```python
from build123d import *

# Parameters (mm, degrees)
F0_R           = 32.5
F0_R_2         = 11.25
F1_DEPTH       = 2
F2_DEPTH       = 2
F3_R           = 32.5
F4_DEPTH       = 2
F6_D           = 3
F6_DEPTH       = 12
F6_CSINK_D     = 6.5
F6_CSINK_ANGLE = 45
F6_TIP         = 0.9012909285


with BuildPart() as f1:
    # F0 (on Top) → F1 (new body)
    with BuildSketch(Plane.XY):
        Circle(F0_R)
        with BuildLine():
            Line((-21.25, 17.4553000547), (-21.25, 21.25))
            Line((-21.25, 21.25), (-17.4553000547, 21.25))
            ThreePointArc((-17.4553000547, 21.25), (0, 27.5), (17.4553000547, 21.25))
            Line((17.4553000547, 21.25), (21.25, 21.25))
            Line((21.25, 21.25), (21.25, 17.4553000547))
            ThreePointArc((21.25, 17.4553000547), (25.8903939715, 9.2702481089), (27.5, 0))
            ThreePointArc((27.5, 0), (25.8903939715, -9.2702481089), (21.25, -17.4553000547))
            Line((21.25, -17.4553000547), (21.25, -21.25))
            Line((21.25, -21.25), (17.4553000547, -21.25))
            ThreePointArc((17.4553000547, -21.25), (0, -27.5), (-17.4553000547, -21.25))
            Line((-17.4553000547, -21.25), (-21.25, -21.25))
            Line((-21.25, -21.25), (-21.25, -17.4553000547))
            ThreePointArc((-21.25, -17.4553000547), (-27.5, 0), (-21.25, 17.4553000547))
        make_face(mode=Mode.SUBTRACT)
        with BuildLine():
            Line((-17.4553000547, 21.25), (-21.25, 21.25))
            Line((-21.25, 21.25), (-21.25, 17.4553000547))
            ThreePointArc((-21.25, 17.4553000547), (-19.4454364826, 19.4454364826), (-17.4553000547, 21.25))
        make_face()
        with BuildLine():
            Line((21.25, 21.25), (17.4553000547, 21.25))
            ThreePointArc((17.4553000547, 21.25), (19.4454364826, 19.4454364826), (21.25, 17.4553000547))
            Line((21.25, 17.4553000547), (21.25, 21.25))
        make_face()
        with BuildLine():
            Line((21.25, -21.25), (21.25, -17.4553000547))
            ThreePointArc((21.25, -17.4553000547), (19.4454364826, -19.4454364826), (17.4553000547, -21.25))
            Line((17.4553000547, -21.25), (21.25, -21.25))
        make_face()
        with BuildLine():
            ThreePointArc((-17.4553000547, -21.25), (-19.4454364826, -19.4454364826), (-21.25, -17.4553000547))
            Line((-21.25, -17.4553000547), (-21.25, -21.25))
            Line((-21.25, -21.25), (-17.4553000547, -21.25))
        make_face()
        with BuildLine():
            Line((17.4553000547, -21.25), (-17.4553000547, -21.25))
            ThreePointArc((-17.4553000547, -21.25), (0, -27.5), (17.4553000547, -21.25))
        make_face()
        with BuildLine():
            ThreePointArc((27.5, 0), (25.8903939715, 9.2702481089), (21.25, 17.4553000547))
            Line((21.25, 17.4553000547), (21.25, -17.4553000547))
            ThreePointArc((21.25, -17.4553000547), (25.8903939715, -9.2702481089), (27.5, 0))
        make_face()
        with BuildLine():
            ThreePointArc((17.4553000547, 21.25), (0, 27.5), (-17.4553000547, 21.25))
            Line((-17.4553000547, 21.25), (17.4553000547, 21.25))
        make_face()
        with BuildLine():
            Line((-21.25, -17.4553000547), (-21.25, 17.4553000547))
            ThreePointArc((-21.25, 17.4553000547), (-27.5, 0), (-21.25, -17.4553000547))
        make_face()
        with BuildLine():
            Line((17.4553000547, 21.25), (-17.4553000547, 21.25))
            ThreePointArc((-17.4553000547, 21.25), (-19.4454364826, 19.4454364826), (-21.25, 17.4553000547))
            Line((-21.25, 17.4553000547), (-21.25, -17.4553000547))
            ThreePointArc((-21.25, -17.4553000547), (-19.4454364826, -19.4454364826), (-17.4553000547, -21.25))
            Line((-17.4553000547, -21.25), (17.4553000547, -21.25))
            ThreePointArc((17.4553000547, -21.25), (19.4454364826, -19.4454364826), (21.25, -17.4553000547))
            Line((21.25, -17.4553000547), (21.25, 17.4553000547))
            ThreePointArc((21.25, 17.4553000547), (19.4454364826, 19.4454364826), (17.4553000547, 21.25))
        make_face()
        Circle(F0_R_2, mode=Mode.SUBTRACT)
    extrude(amount=F1_DEPTH)

    # F0 (on Top) → F2 (join)
    with BuildSketch(Plane.XY):
        Circle(F0_R)
        with BuildLine():
            Line((-21.25, 17.4553000547), (-21.25, 21.25))
            Line((-21.25, 21.25), (-17.4553000547, 21.25))
            ThreePointArc((-17.4553000547, 21.25), (0, 27.5), (17.4553000547, 21.25))
            Line((17.4553000547, 21.25), (21.25, 21.25))
            Line((21.25, 21.25), (21.25, 17.4553000547))
            ThreePointArc((21.25, 17.4553000547), (25.8903939715, 9.2702481089), (27.5, 0))
            ThreePointArc((27.5, 0), (25.8903939715, -9.2702481089), (21.25, -17.4553000547))
            Line((21.25, -17.4553000547), (21.25, -21.25))
            Line((21.25, -21.25), (17.4553000547, -21.25))
            ThreePointArc((17.4553000547, -21.25), (0, -27.5), (-17.4553000547, -21.25))
            Line((-17.4553000547, -21.25), (-21.25, -21.25))
            Line((-21.25, -21.25), (-21.25, -17.4553000547))
            ThreePointArc((-21.25, -17.4553000547), (-27.5, 0), (-21.25, 17.4553000547))
        make_face(mode=Mode.SUBTRACT)
        with BuildLine():
            Line((-21.25, -17.4553000547), (-21.25, 17.4553000547))
            ThreePointArc((-21.25, 17.4553000547), (-27.5, 0), (-21.25, -17.4553000547))
        make_face()
        with BuildLine():
            Line((17.4553000547, -21.25), (-17.4553000547, -21.25))
            ThreePointArc((-17.4553000547, -21.25), (0, -27.5), (17.4553000547, -21.25))
        make_face()
        with BuildLine():
            ThreePointArc((27.5, 0), (25.8903939715, 9.2702481089), (21.25, 17.4553000547))
            Line((21.25, 17.4553000547), (21.25, -17.4553000547))
            ThreePointArc((21.25, -17.4553000547), (25.8903939715, -9.2702481089), (27.5, 0))
        make_face()
        with BuildLine():
            ThreePointArc((17.4553000547, 21.25), (0, 27.5), (-17.4553000547, 21.25))
            Line((-17.4553000547, 21.25), (17.4553000547, 21.25))
        make_face()
        with BuildLine():
            ThreePointArc((-17.4553000547, -21.25), (-19.4454364826, -19.4454364826), (-21.25, -17.4553000547))
            Line((-21.25, -17.4553000547), (-21.25, -21.25))
            Line((-21.25, -21.25), (-17.4553000547, -21.25))
        make_face()
        with BuildLine():
            Line((21.25, -21.25), (21.25, -17.4553000547))
            ThreePointArc((21.25, -17.4553000547), (19.4454364826, -19.4454364826), (17.4553000547, -21.25))
            Line((17.4553000547, -21.25), (21.25, -21.25))
        make_face()
        with BuildLine():
            Line((21.25, 21.25), (17.4553000547, 21.25))
            ThreePointArc((17.4553000547, 21.25), (19.4454364826, 19.4454364826), (21.25, 17.4553000547))
            Line((21.25, 17.4553000547), (21.25, 21.25))
        make_face()
        with BuildLine():
            Line((-17.4553000547, 21.25), (-21.25, 21.25))
            Line((-21.25, 21.25), (-21.25, 17.4553000547))
            ThreePointArc((-21.25, 17.4553000547), (-19.4454364826, 19.4454364826), (-17.4553000547, 21.25))
        make_face()
    extrude(amount=-F2_DEPTH)

    # F3 (on face) → F4 (join)
    with BuildSketch(Plane.XY.offset(2)):
        Circle(F3_R)
        with BuildLine():
            ThreePointArc((-7.9549512883, 7.9549512883), (0, 11.25), (7.9549512883, 7.9549512883))
            ThreePointArc((7.9549512883, 7.9549512883), (10.3936447408, 4.3051886141), (11.25, 0))
            ThreePointArc((11.25, 0), (10.3936447408, -4.3051886141), (7.9549512883, -7.9549512883))
            ThreePointArc((7.9549512883, -7.9549512883), (0, -11.25), (-7.9549512883, -7.9549512883))
            ThreePointArc((-7.9549512883, -7.9549512883), (-11.25, 0), (-7.9549512883, 7.9549512883))
        make_face(mode=Mode.SUBTRACT)
        with BuildLine():
            ThreePointArc((-2.1213203436, 2.1213203436), (0, 3), (2.1213203436, 2.1213203436))
            Line((2.1213203436, 2.1213203436), (7.9549512883, 7.9549512883))
            ThreePointArc((7.9549512883, 7.9549512883), (0, 11.25), (-7.9549512883, 7.9549512883))
            Line((-7.9549512883, 7.9549512883), (-2.1213203436, 2.1213203436))
        make_face()
        with BuildLine():
            ThreePointArc((-2.1213203436, -2.1213203436), (-3, 0), (-2.1213203436, 2.1213203436))
            Line((-2.1213203436, 2.1213203436), (-7.9549512883, 7.9549512883))
            ThreePointArc((-7.9549512883, 7.9549512883), (-11.25, 0), (-7.9549512883, -7.9549512883))
            Line((-7.9549512883, -7.9549512883), (-2.1213203436, -2.1213203436))
        make_face()
        with BuildLine():
            Line((7.9549512883, -7.9549512883), (2.1213203436, -2.1213203436))
            ThreePointArc((2.1213203436, -2.1213203436), (0, -3), (-2.1213203436, -2.1213203436))
            Line((-2.1213203436, -2.1213203436), (-7.9549512883, -7.9549512883))
            ThreePointArc((-7.9549512883, -7.9549512883), (0, -11.25), (7.9549512883, -7.9549512883))
        make_face()
        with BuildLine():
            ThreePointArc((2.1213203436, 2.1213203436), (2.7716385975, 1.1480502971), (3, 0))
            ThreePointArc((3, 0), (2.7716385975, -1.1480502971), (2.1213203436, -2.1213203436))
            Line((2.1213203436, -2.1213203436), (7.9549512883, -7.9549512883))
            ThreePointArc((7.9549512883, -7.9549512883), (10.3936447408, -4.3051886141), (11.25, 0))
            ThreePointArc((11.25, 0), (10.3936447408, 4.3051886141), (7.9549512883, 7.9549512883))
            Line((7.9549512883, 7.9549512883), (2.1213203436, 2.1213203436))
        make_face()
    extrude(amount=F4_DEPTH)

    # F6
    with Locations(Plane.XY.offset(4)):
        with Locations((-15.7731351997, 15.1271263808), (-15.7731351997, -15.8728736192), (15.2268648003, -15.8728736192), (15.2268648003, 15.1271263808)):
            CounterSinkHole(F6_D / 2, F6_CSINK_D / 2, depth=F6_DEPTH, counter_sink_angle=F6_CSINK_ANGLE)
            with Locations((0, 0, -(F6_DEPTH + F6_TIP / 2))):  # 118° drill point
                Cone(0, F6_D / 2, F6_TIP, mode=Mode.SUBTRACT)


solid = f1.part
```
Build history of the part. All positions in model axes, mm. A direction names the side the tool comes from. Coordinates: 2 decimals unless noted, no trailing zeros. Order: outer loops, then holes, each group sorted by start corner. A loop starts at its lowest first (then second) coordinate and runs counter-clockwise, first axis right, second up. Notation, with made-up numbers: (65.25, 66) -> (101.25, 66) arc R29 cw to (101.25, 102) -> close; hole circle Ø10 at (66, -25). An arc over 180 degrees is marked (long way). Answer in a Markdown table with one row per item. Add a question column.
Q1. Which spindle directions (+Z, -Z, +X, -X, +Y, -Y) get a long thin tool onto all of the face, cutting with end or side? Do faces 4 (the face through (17.267, -15.783, 1.083)), 5 (the face through (19.47, -19.42, -0.99)). Say none if no direction does.
Q2. Mould opens along X. For faces 1 (the face through (31, 9.76, 0.96)), 2 (the face through (7, 0, 4)), 3 (the face through (5.19, -9.98, 0.99)) say: +X half, -X half, draft (parallel to the pull), parting line (faces both ways), or undercut.
Q3. Band-saw the part on A-A, the plane x = 0. List the corners of the cut face in (y, z), then the cut area to 3 significant figures.
Q4. Drop flat-ended pins along their axis: pin 1 (20 mm diameter, centred on x = 0, y = 0, fed in from +Z); pin 2 (6 mm diameter, centred on x = -16.5, y = -2.5, fed in from -Z); pin 3 (1.5 mm diameter, centred on x = -1.5, y = 5, fed in from -Z); pin 4 (1 mm diameter, centred on x = -4, z = -1, fed in from -Y). Give the stop position or say it passes through.
Q5. Wall check: line 1 along Y through (x, z) = (0, 1); line 2 along Z through (x, y) = (-3, -16); line 3 along X through (y, z) = (-2.5, 2.95). Give the ranges that are in metal, low to high. Write a range as [from, to].
Q6. Band-saw the part on B-B, the plane z = 0.9. List the corners of the cut face in (x, y).
Answers follow:
| question | item | result |
|---|---|---|
| 1 | face 4 | +Z |
| 1 | face 5 | -Z |
| 2 | face 1 | parting line |
| 2 | face 2 | draft |
| 2 | face 3 | undercut |
| 3 | outline | (-32.5, -2) -> (-21.25, -2) -> (-21.25, 0) -> (-11.25, 0) -> (-11.25, 2) -> (-3, 2) -> (-3, 4) -> (-32.5, 4) -> close; (3, 2) -> (11.25, 2) -> (11.25, 0) -> (21.25, 0) -> (21.25, -2) -> (32.5, -2) -> (32.5, 4) -> (3, 4) -> close |
| 3 | area | 248 mm^2 |
| 4 | pin 1 | z = 4 |
| 4 | pin 2 | z = 0 |
| 4 | pin 3 | z = 2 |
| 4 | pin 4 | y = -32.31 |
| 5 | line 1 | [-32.5, -11.25], [11.25, 32.5] |
| 5 | line 2 | [0, 4] |
| 5 | line 3 | [-32.4, -1.66], [1.66, 32.4] |
| 6 | outline | circle Ø65 at (0, 0); hole circle Ø3.93 at (-15.77, -15.87); hole circle Ø3.93 at (-15.77, 15.13); hole circle Ø22.5 at (0, 0); hole circle Ø3.93 at (15.23, -15.87); hole circle Ø3.93 at (15.23, 15.13) |
